from build123d import *

# Parameters (mm, degrees)
SKETCH_1_W          = 190
SKETCH_1_H          = 130
SKETCH_1_R          = 2.15
EXTRUDE_1_DEPTH     = 2
FILLET_1_R          = 8
SKETCH_2_R          = 25
CUT_EXTRUDE_1_DEPTH = 10
CUT_EXTRUDE_2_DEPTH = 10
FILLET_2_R          = 2
SKETCH_5_R          = 1.65
CUT_EXTRUDE_5_DEPTH = 3.3
SKETCH_6_R          = 1.65
CUT_EXTRUDE_6_DEPTH = 3.3
SKETCH_7_R          = 2.15
CUT_EXTRUDE_7_DEPTH = 3.3


with BuildPart() as part:
    # 草图1 → 凸台-拉伸1 (new body)
    with BuildSketch(Plane.XY):
        with Locations((95, 65)):
            Rectangle(SKETCH_1_W, SKETCH_1_H)
        with Locations((136.4, 7.5)):
            Circle(SKETCH_1_R, mode=Mode.SUBTRACT)
        with Locations((185, 15.5)):
            Circle(SKETCH_1_R, mode=Mode.SUBTRACT)
        with Locations((185, 114.5)):
            Circle(SKETCH_1_R, mode=Mode.SUBTRACT)
        with Locations((136.4, 114.5)):
            Circle(SKETCH_1_R, mode=Mode.SUBTRACT)
        with Locations((136.4, 122.5)):
            Circle(SKETCH_1_R, mode=Mode.SUBTRACT)
        with Locations((185, 122.5)):
            Circle(SKETCH_1_R, mode=Mode.SUBTRACT)
        with Locations((5, 122.5)):
            Circle(SKETCH_1_R, mode=Mode.SUBTRACT)
        with Locations((5, 114.5)):
            Circle(SKETCH_1_R, mode=Mode.SUBTRACT)
        with Locations((5, 15.5)):
            Circle(SKETCH_1_R, mode=Mode.SUBTRACT)
        with Locations((53.6, 15.5)):
            Circle(SKETCH_1_R, mode=Mode.SUBTRACT)
        with Locations((53.6, 7.5)):
            Circle(SKETCH_1_R, mode=Mode.SUBTRACT)
        with Locations((5, 7.5)):
            Circle(SKETCH_1_R, mode=Mode.SUBTRACT)
        with Locations((53.6, 122.5)):
            Circle(SKETCH_1_R, mode=Mode.SUBTRACT)
        with Locations((53.6, 114.5)):
            Circle(SKETCH_1_R, mode=Mode.SUBTRACT)
        with Locations((185, 7.5)):
            Circle(SKETCH_1_R, mode=Mode.SUBTRACT)
        with Locations((136.4, 15.5)):
            Circle(SKETCH_1_R, mode=Mode.SUBTRACT)
    extrude(amount=EXTRUDE_1_DEPTH)

    # 圆角1
    fillet_1_edges = [part.edges().sort_by_distance(p)[0] for p in [
        (0, 0, 1),
        (0, 130, 1),
        (190, 130, 1),
        (190, 0, 1),
    ]]
    fillet(fillet_1_edges, radius=FILLET_1_R)

    # 草图2 → 切除-拉伸1 (cut)
    with BuildSketch(Plane(origin=(0, 0, 0), x_dir=(-1, 0, 0), z_dir=(0, 0, -1))):
        with Locations((-95, 65)):
            Circle(SKETCH_2_R)
        with BuildLine():
            Line((-21, 85), (-14, 85))
            ThreePointArc((-14, 85), (-11.171572875, 86.171572875), (-10, 89))
            Line((-10, 89), (-10, 96))
            ThreePointArc((-10, 96), (-11.171572875, 98.828427125), (-14, 100))
            Line((-14, 100), (-21, 100))
            ThreePointArc((-21, 100), (-23.828427125, 98.828427125), (-25, 96))
            Line((-25, 96), (-25, 89))
            ThreePointArc((-25, 89), (-23.828427125, 86.171572875), (-21, 85))
        make_face()
        with BuildLine():
            Line((-21, 30), (-14, 30))
            ThreePointArc((-14, 30), (-11.171572875, 31.171572875), (-10, 34))
            Line((-10, 34), (-10, 41))
            ThreePointArc((-10, 41), (-11.171572875, 43.828427125), (-14, 45))
            Line((-14, 45), (-21, 45))
            ThreePointArc((-21, 45), (-23.828427125, 43.828427125), (-25, 41))
            Line((-25, 41), (-25, 34))
            ThreePointArc((-25, 34), (-23.828427125, 31.171572875), (-21, 30))
        make_face()
        with BuildLine():
            Line((-165, 96), (-165, 89))
            ThreePointArc((-165, 89), (-166.171572875, 86.171572875), (-169, 85))
            Line((-169, 85), (-176, 85))
            ThreePointArc((-176, 85), (-178.828427125, 86.171572875), (-180, 89))
            Line((-180, 89), (-180, 96))
            ThreePointArc((-180, 96), (-178.828427125, 98.828427125), (-176, 100))
            Line((-176, 100), (-169, 100))
            ThreePointArc((-169, 100), (-166.171572875, 98.828427125), (-165, 96))
        make_face()
        with BuildLine():
            Line((-169, 45), (-176, 45))
            ThreePointArc((-176, 45), (-178.828427125, 43.828427125), (-180, 41))
            Line((-180, 41), (-180, 34))
            ThreePointArc((-180, 34), (-178.828427125, 31.171572875), (-176, 30))
            Line((-176, 30), (-169, 30))
            ThreePointArc((-169, 30), (-166.171572875, 31.171572875), (-165, 34))
            Line((-165, 34), (-165, 41))
            ThreePointArc((-165, 41), (-166.171572875, 43.828427125), (-169, 45))
        make_face()
    extrude(amount=-CUT_EXTRUDE_1_DEPTH, mode=Mode.SUBTRACT)

    # 草图4 → 切除-拉伸2 (cut)
    with BuildSketch(Plane(origin=(0, 0, 0), x_dir=(-1, 0, 0), z_dir=(0, 0, -1))):
        with BuildLine():
            Line((-40, 55), (-17.087121525, 65))
            Line((-17.087121525, 65), (-40, 75))
            Line((-40, 75), (-40, 66.65))
            Line((-40, 66.65), (-60, 66.65))
            ThreePointArc((-60, 66.65), (-61.65, 65), (-60, 63.35))
            Line((-60, 63.35), (-40, 63.35))
            Line((-40, 63.35), (-40, 55))
        make_face()
    extrude(amount=-CUT_EXTRUDE_2_DEPTH, mode=Mode.SUBTRACT)

    # 圆角2
    fillet_2_edges = [part.edges().sort_by_distance(p)[0] for p in [
        (40, 66.65, 1),
        (40, 75, 1),
        (17.087121525, 65, 1),
        (40, 55, 1),
        (40, 63.35, 1),
    ]]
    fillet(fillet_2_edges, radius=FILLET_2_R)

    # 草图5 → 切除-拉伸5 (cut)
    with BuildSketch(Plane(origin=(0, 0, 0), x_dir=(-1, 0, 0), z_dir=(0, 0, -1))):
        with Locations((-160, 35)):
            Circle(SKETCH_5_R)
        with Locations((-185, 95)):
            Circle(SKETCH_5_R)
        with Locations((-185, 35)):
            Circle(SKETCH_5_R)
        with Locations((-160, 95)):
            Circle(SKETCH_5_R)
    cut_extrude_5 = extrude(amount=-CUT_EXTRUDE_5_DEPTH, mode=Mode.SUBTRACT)

    # 草图6 → 切除-拉伸6 (cut)
    with BuildSketch(Plane(origin=(0, 0, 0), x_dir=(-1, 0, 0), z_dir=(0, 0, -1))):
        with Locations((-140, 35)):
            Circle(SKETCH_6_R)
        with Locations((-130, 35)):
            Circle(SKETCH_6_R)
        with Locations((-130, 50)):
            Circle(SKETCH_6_R)
        with Locations((-130, 65)):
            Circle(SKETCH_6_R)
        with Locations((-130, 80)):
            Circle(SKETCH_6_R)
        with Locations((-130, 95)):
            Circle(SKETCH_6_R)
        with Locations((-140, 50)):
            Circle(SKETCH_6_R)
        with Locations((-140, 65)):
            Circle(SKETCH_6_R)
        with Locations((-140, 80)):
            Circle(SKETCH_6_R)
        with Locations((-140, 95)):
            Circle(SKETCH_6_R)
        with Locations((-95, 30)):
            Circle(SKETCH_6_R)
        with Locations((-119.748737342, 40.251262658)):
            Circle(SKETCH_6_R)
        with Locations((-119.748737342, 89.748737342)):
            Circle(SKETCH_6_R)
        with Locations((-95, 100)):
            Circle(SKETCH_6_R)
        with Locations((-70.251262658, 89.748737342)):
            Circle(SKETCH_6_R)
        with Locations((-70.251262658, 40.251262658)):
            Circle(SKETCH_6_R)
    cut_extrude_6 = extrude(amount=-CUT_EXTRUDE_6_DEPTH, mode=Mode.SUBTRACT)

    # 镜向1: 切除-拉伸6 across plane
    add(cut_extrude_6.mirror(Plane.ZY.offset(-95)), mode=Mode.SUBTRACT)

    # 镜向2: 切除-拉伸5 across plane
    add(cut_extrude_5.mirror(Plane.ZY.offset(-95)), mode=Mode.SUBTRACT)

    # 草图7 → 切除-拉伸7 (cut)
    with BuildSketch(Plane.XY.offset(2)):
        with Locations((45, 37)):
            Circle(SKETCH_7_R)
        with Locations((45, 93)):
            Circle(SKETCH_7_R)
    extrude(amount=-CUT_EXTRUDE_7_DEPTH, mode=Mode.SUBTRACT)


solid = part.part
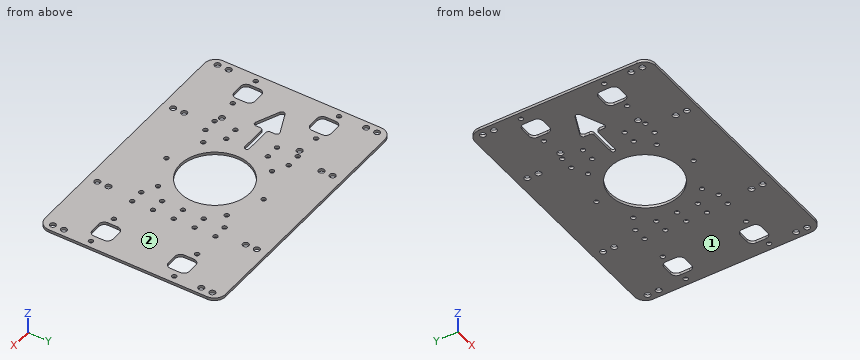
Verification items for the finished model (mm, model axes). Face numbers are marked on the shaded views. Coordinates: 2 decimals unless noted, no trailing zeros. Order: outer loops, then holes, each group sorted by start corner. A loop starts at its lowest first (then second) coordinate and runs counter-clockwise, first axis right, second up. Notation, with made-up numbers: (84, 56) -> (143, 56) arc R31 ccw to (143, 93) -> close; hole circle Ø1 at (25, 40.25). An arc over 180 degrees is marked (long way). Use CSV: the item, a comma, the result in double quotes. Start each with the question number.
Q1. Thickness scan on line 1 along Y through (x, z) = (14.5, 0.45); line 2 along Y through (x, z) = (130, 1.55); line 3 along Y through (x, z) = (95, 1.45). Record the ranges inside material, lowest first.
Q2. Draft check along Z on the marked faces 1 and 2. Enter one of: +Z half, -Z half, draft (parallel to the pull), parting line (faces both ways), or undercut.
Q3. Section check A-A, the plane x = 103. Record the cut outline in (y, z), and give its area (3 significant figures).
Q4. Section check B-B, the plane z = 1.35. Give the number of separate pieces and of enclosed holes in the cut face, and give its area (3 significant figures).
Q5. Depth check by flat-ended pin: P1, Ø4, axis at x = 73, y = 46, coming from the -Z side; P2, Ø2.5, axis at x = 50, y = 35, coming from the +Z side. Enter the tip coordinate at first touch or a pass-through.
Returned:
1,line 1,"y = 0 to 30, 45 to 85, 100 to 130"
1,line 2,"y = 0 to 33.35, 36.65 to 48.35, 51.65 to 63.35, 66.65 to 78.35, 81.65 to 93.35, 96.65 to 130"
1,line 3,"y = 0 to 28.35, 31.65 to 40, 90 to 98.35, 101.65 to 130"
2,face 1,"-Z half"
2,face 2,"+Z half"
3,outline,"(0, 0) -> (41.31, 0) -> (41.31, 2) -> (0, 2) -> close; (88.69, 0) -> (130, 0) -> (130, 2) -> (88.69, 2) -> close"
3,area,"165 mm^2"
4,separate pieces,"1"
4,enclosed holes,"56"
4,area,"21,000 mm^2"
5,P1,"stops at z = 0"
5,P2,"passes through"
